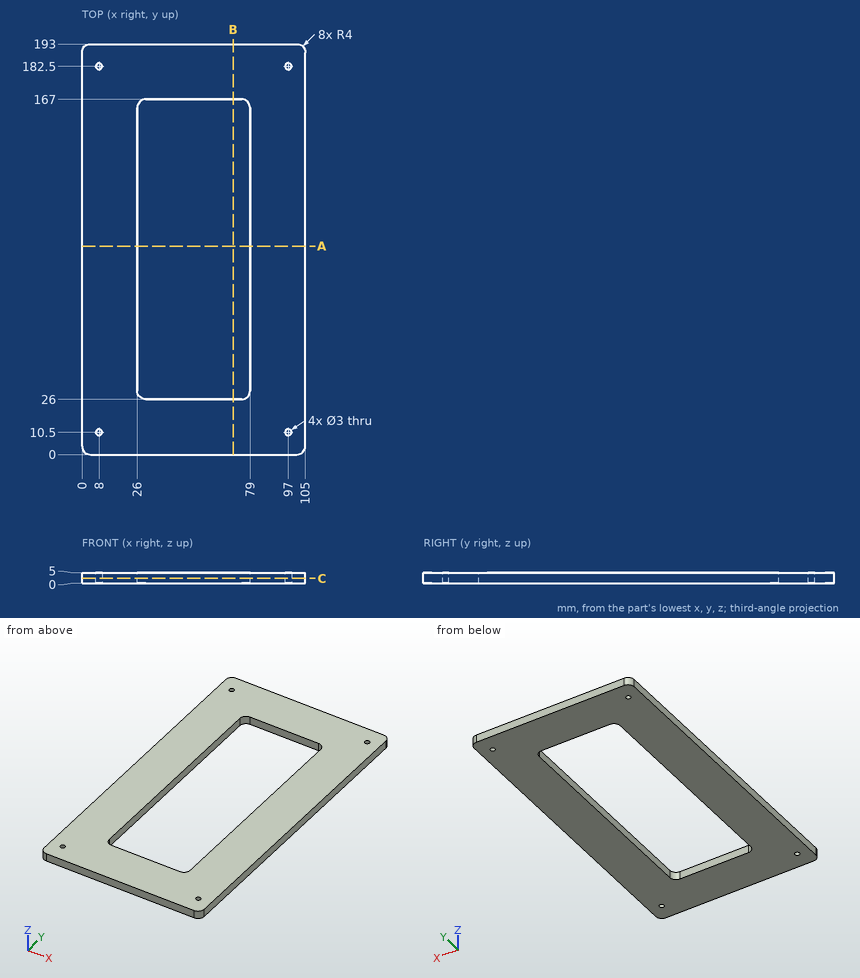
Geometry: see drawing. Coordinates: mm, zero at the bounding-box minimum. Give positions to 0.01 mm unless a question says otherwise; leave off trailing zeros. Loops run counter-clockwise (first coordinate to the right, second up) from the corner with the lowest first, then second, coordinate; pieces in that order, holes last. Notation, with made-up numbers: (82.25, -20.5) -> (112.25, -20.5) arc R30 ccw to (112.25, 9.5) -> close; hole circle Ø4 at (58, 0.5). An arc over 180 degrees is marked (long way). Answer as a JSON object with one key per item and string values. Group by question number.
Item 1: Line query: probe 1 along Y at (x, z) = (8, 1.7); probe 2 along X at (y, z) = (182.5, 3); probe 3 along X at (y, z) = (90, 3.4). Output: solid intervals per line, ascending.
Item 2: Cut plane C-C, the plane z = 2.25. Return the cut outline in (x, y), and give its area (3 significant figures).
Item 3: Cut plane A-A, the plane y = 98. Return the cut outline in (x, z), and give its area (3 significant figures).
Item 4: Cut plane B-B, the plane x = 71. Return the cut outline in (y, z).
Checks:
{
 "1": {"probe 1": "y = 0 to 9, 12 to 181, 184 to 193", "probe 2": "x = 0 to 6.5, 9.5 to 95.5, 98.5 to 105", "probe 3": "x = 0 to 26, 79 to 105"},
 "2": {"outline": "(0, 4) arc R4 ccw to (4, 0) -> (101, 0) arc R4 ccw to (105, 4) -> (105, 189) arc R4 ccw to (101, 193) -> (4, 193) arc R4 ccw to (0, 189) -> close; hole circle Ø3 at (8, 10.5); hole circle Ø3 at (8, 182.5); hole (26, 30) arc R4 ccw to (30, 26) -> (75, 26) arc R4 ccw to (79, 30) -> (79, 163) arc R4 ccw to (75, 167) -> (30, 167) arc R4 ccw to (26, 163) -> close; hole circle Ø3 at (97, 10.5); hole circle Ø3 at (97, 182.5)", "area": "12,800 mm²"},
 "3": {"outline": "(0, 0) -> (26, 0) -> (26, 5) -> (0, 5) -> close; (79, 0) -> (105, 0) -> (105, 5) -> (79, 5) -> close", "area": "260 mm²"},
 "4": {"outline": "(0, 0) -> (26, 0) -> (26, 5) -> (0, 5) -> close; (167, 0) -> (193, 0) -> (193, 5) -> (167, 5) -> close"}
}
